```python
from build123d import *

# Parameters (mm, degrees)
SKETCH1_W               = 212.5
SKETCH1_H               = 339.725
BOSS_EXTRUDE1_DEPTH     = 6
SKETCH2_W               = 6.5
SKETCH2_H               = 20
BOSS_EXTRUDE2_DEPTH     = 24
CUT_EXTRUDE1_DEPTH      = 393.36344838
CUT_EXTRUDE1_DEPTH_BACK = 393.36344838
SKETCH3_R               = 4
FILLET2_R               = 5
SKETCH5_R               = 3.175
CUT_EXTRUDE2_DEPTH      = 402.314497153


with BuildPart() as part:
    # Sketch1 → Boss-Extrude1 (new body)
    with BuildSketch(Plane.XY):
        with Locations((106.25, -169.8625)):
            Rectangle(SKETCH1_W, SKETCH1_H)
    extrude(amount=BOSS_EXTRUDE1_DEPTH)

    # Sketch2 → Boss-Extrude2 (add)
    with BuildSketch(Plane.XY.offset(6)):
        with Locations((21.75, -35.2425)):
            Rectangle(SKETCH2_W, SKETCH2_H)
        with Locations((50.75, -35.2425)):
            Rectangle(SKETCH2_W, SKETCH2_H)
        with Locations((190.75, -35.2425)):
            Rectangle(SKETCH2_W, SKETCH2_H)
        with Locations((161.75, -35.2425)):
            Rectangle(SKETCH2_W, SKETCH2_H)
        with Locations((133.75, -104.5325)):
            Rectangle(SKETCH2_W, SKETCH2_H)
        with Locations((165.25, -104.5325)):
            Rectangle(SKETCH2_W, SKETCH2_H)
        with Locations((165.25, -235.1925)):
            Rectangle(SKETCH2_W, SKETCH2_H)
        with Locations((21.75, -304.4825)):
            Rectangle(SKETCH2_W, SKETCH2_H)
        with Locations((50.75, -304.4825)):
            Rectangle(SKETCH2_W, SKETCH2_H)
        with Locations((190.75, -304.4825)):
            Rectangle(SKETCH2_W, SKETCH2_H)
        with Locations((161.75, -304.4825)):
            Rectangle(SKETCH2_W, SKETCH2_H)
        with Locations((133.75, -235.1925)):
            Rectangle(SKETCH2_W, SKETCH2_H)
    extrude(amount=BOSS_EXTRUDE2_DEPTH)

    # Sketch3 → Cut-Extrude1 (cut, two sides: drawn at the far end of the back side and taken through both)
    with BuildSketch(Plane.ZY.offset(-18.5).offset(-CUT_EXTRUDE1_DEPTH_BACK)):
        with Locations(Location((18, -35.2425, 0), (0, 0, 180))):
            Circle(SKETCH3_R)
        with Locations((18, -235.1925)):
            Circle(SKETCH3_R)
        with Locations(Location((18, -304.4825, 0), (0, 0, 270))):
            Circle(SKETCH3_R)
        with Locations(Location((18, -104.5325, 0), (0, 0, 180))):
            Circle(SKETCH3_R)
        with BuildLine():
            Line((18, -25.2425), (18, -12.982943413))
            Line((18, -12.982943413), (51.949532367, -12.982943413))
            Line((51.949532367, -12.982943413), (51.949532367, -57.481006387))
            Line((51.949532367, -57.481006387), (18, -57.481006387))
            Line((18, -57.481006387), (18, -45.2425))
            ThreePointArc((18, -45.2425), (28, -35.2425), (18, -25.2425))
        make_face()
        with BuildLine():
            Line((52.442304634, -132.399123951), (18, -132.399123951))
            Line((18, -132.399123951), (18, -114.5325))
            ThreePointArc((18, -114.5325), (28, -104.5325), (18, -94.5325))
            Line((18, -94.5325), (18, -71.59149594))
            Line((18, -71.59149594), (52.442304634, -71.59149594))
            Line((52.442304634, -71.59149594), (52.442304634, -132.399123951))
        make_face()
        with BuildLine():
            Line((52.599532243, -270.375386727), (18, -270.375386727))
            Line((18, -270.375386727), (18, -245.1925))
            ThreePointArc((18, -245.1925), (28, -235.1925), (18, -225.1925))
            Line((18, -225.1925), (18, -207.306351849))
            Line((18, -207.306351849), (52.599532243, -207.306351849))
            Line((52.599532243, -207.306351849), (52.599532243, -270.375386727))
        make_face()
        with BuildLine():
            Line((52.621034016, -326.721115515), (18, -326.721115515))
            Line((18, -326.721115515), (18, -314.4825))
            ThreePointArc((18, -314.4825), (28, -304.4825), (18, -294.4825))
            Line((18, -294.4825), (18, -282.222834285))
            Line((18, -282.222834285), (52.621034016, -282.222834285))
            Line((52.621034016, -282.222834285), (52.621034016, -326.721115515))
        make_face()
    extrude(amount=CUT_EXTRUDE1_DEPTH + CUT_EXTRUDE1_DEPTH_BACK, mode=Mode.SUBTRACT)

    # Fillet2
    fillet2_edges = [part.edges().sort_by_distance(p)[0] for p in [
        (190.75, -45.2425, 6),
        (194, -35.2425, 6),
        (190.75, -25.2425, 6),
        (50.75, -45.2425, 6),
        (54, -35.2425, 6),
        (50.75, -25.2425, 6),
        (21.75, -25.2425, 6),
        (18.5, -35.2425, 6),
        (21.75, -45.2425, 6),
        (161.75, -25.2425, 6),
        (158.5, -35.2425, 6),
        (161.75, -45.2425, 6),
        (161.75, -294.4825, 6),
        (161.75, -314.4825, 6),
        (158.5, -304.4825, 6),
        (190.75, -314.4825, 6),
        (194, -304.4825, 6),
        (190.75, -294.4825, 6),
        (165.25, -245.1925, 6),
        (168.5, -235.1925, 6),
        (165.25, -225.1925, 6),
        (133.75, -225.1925, 6),
        (130.5, -235.1925, 6),
        (133.75, -245.1925, 6),
        (50.75, -314.4825, 6),
        (54, -304.4825, 6),
        (50.75, -294.4825, 6),
        (21.75, -294.4825, 6),
        (21.75, -314.4825, 6),
        (18.5, -304.4825, 6),
        (165.25, -114.5325, 6),
        (165.25, -94.5325, 6),
        (168.5, -104.5325, 6),
        (133.75, -94.5325, 6),
        (130.5, -104.5325, 6),
        (133.75, -114.5325, 6),
    ]]
    fillet(fillet2_edges, radius=FILLET2_R)

    # Sketch5 → Cut-Extrude2 (cut, through all)
    with BuildSketch(Plane.XY.offset(6)):
        with BuildLine():
            Line((141, -10), (86.089952747, -10))
            ThreePointArc((86.089952747, -10), (83.699567237, -11.767840789), (84.689838532, -14.571154312))
            Line((84.689838532, -14.571154312), (139.599885785, -51.690714779))
            ThreePointArc((139.599885785, -51.690714779), (142.172543061, -51.827533014), (143.5, -49.619560467))
            Line((143.5, -49.619560467), (143.5, -12.5))
            ThreePointArc((143.5, -12.5), (142.767766953, -10.732233047), (141, -10))
        make_face()
        with BuildLine():
            ThreePointArc((0, -12.7), (3.719743879, -3.719743879), (12.7, 0))
            Line((12.7, 0), (0, 0))
            Line((0, 0), (0, -12.7))
        make_face()
        with BuildLine():
            Line((212.5, 0), (199.8, 0))
            ThreePointArc((199.8, 0), (208.780256121, -3.719743879), (212.5, -12.7))
            Line((212.5, -12.7), (212.5, 0))
        make_face()
        with BuildLine():
            ThreePointArc((5, -70.4825), (1.464466094, -69.018033906), (0, -65.4825))
            Line((0, -65.4825), (0, -274.2425))
            ThreePointArc((0, -274.2425), (1.464466094, -270.706966094), (5, -269.2425))
            Line((5, -269.2425), (101.25, -269.2425))
            ThreePointArc((101.25, -269.2425), (104.785533906, -267.778033906), (106.25, -264.2425))
            Line((106.25, -264.2425), (106.25, -204.9525))
            ThreePointArc((106.25, -204.9525), (107.714466094, -201.416966094), (111.25, -199.9525))
            Line((111.25, -199.9525), (187.26, -199.9525))
            ThreePointArc((187.26, -199.9525), (190.795533906, -198.488033906), (192.26, -194.9525))
            Line((192.26, -194.9525), (192.26, -144.7725))
            ThreePointArc((192.26, -144.7725), (190.795533906, -141.236966094), (187.26, -139.7725))
            Line((187.26, -139.7725), (111.25, -139.7725))
            ThreePointArc((111.25, -139.7725), (107.714466094, -138.308033906), (106.25, -134.7725))
            Line((106.25, -134.7725), (106.25, -75.4825))
            ThreePointArc((106.25, -75.4825), (104.785533906, -71.946966094), (101.25, -70.4825))
            Line((101.25, -70.4825), (5, -70.4825))
        make_face()
        with BuildLine():
            Line((212.5, -339.725), (212.5, -327.025))
            ThreePointArc((212.5, -327.025), (208.780256121, -336.005256121), (199.8, -339.725))
            Line((199.8, -339.725), (212.5, -339.725))
        make_face()
        with BuildLine():
            Line((0, -339.725), (12.7, -339.725))
            ThreePointArc((12.7, -339.725), (3.719743879, -336.005256121), (0, -327.025))
            Line((0, -327.025), (0, -339.725))
        make_face()
        with BuildLine():
            ThreePointArc((72.900114215, -18.671785221), (70.327456939, -18.534966986), (69, -20.742939533))
            Line((69, -20.742939533), (69, -57.8625))
            ThreePointArc((69, -57.8625), (69.732233047, -59.630266953), (71.5, -60.3625))
            Line((71.5, -60.3625), (126.410047253, -60.3625))
            ThreePointArc((126.410047253, -60.3625), (128.800432763, -58.594659211), (127.810161468, -55.791345688))
            Line((127.810161468, -55.791345688), (72.900114215, -18.671785221))
        make_face()
        with BuildLine():
            Line((126.410047253, -279.3625), (71.5, -279.3625))
            ThreePointArc((71.5, -279.3625), (69.732233047, -280.094733047), (69, -281.8625))
            Line((69, -281.8625), (69, -318.982060467))
            ThreePointArc((69, -318.982060467), (70.327456939, -321.190033014), (72.900114215, -321.053214779))
            Line((72.900114215, -321.053214779), (127.810161468, -283.933654312))
            ThreePointArc((127.810161468, -283.933654312), (128.800432763, -281.130340789), (126.410047253, -279.3625))
        make_face()
        with BuildLine():
            Line((139.599885785, -288.034285221), (84.689838532, -325.153845688))
            ThreePointArc((84.689838532, -325.153845688), (83.699567237, -327.957159211), (86.089952747, -329.725))
            Line((86.089952747, -329.725), (141, -329.725))
            ThreePointArc((141, -329.725), (142.767766953, -328.992766953), (143.5, -327.225))
            Line((143.5, -327.225), (143.5, -290.105439533))
            ThreePointArc((143.5, -290.105439533), (142.172543061, -287.897466986), (139.599885785, -288.034285221))
        make_face()
        with Locations((12.7, -12.7)):
            Circle(SKETCH5_R)
        with Locations((199.8, -12.7)):
            Circle(SKETCH5_R)
        with Locations((12.7, -327.025)):
            Circle(SKETCH5_R)
        with Locations((199.8, -327.025)):
            Circle(SKETCH5_R)
    extrude(amount=-CUT_EXTRUDE2_DEPTH, mode=Mode.SUBTRACT)


solid = part.part
```
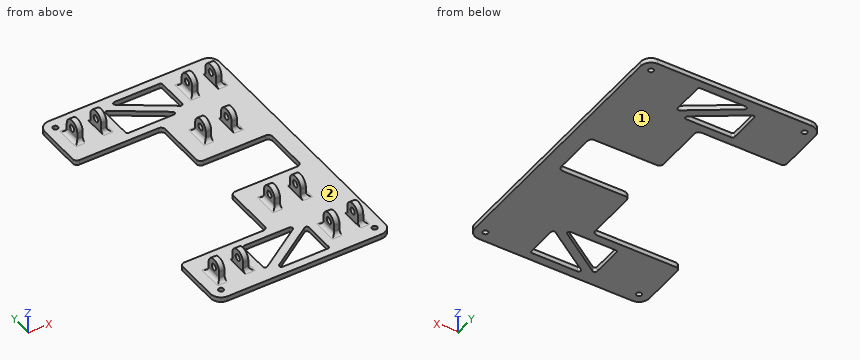
For this review, take the finished solid that the model builds, in its own axes (mm). Face numbers are marked on the shaded views. Round coordinates to 2 decimals unless told otherwise and drop trailing zeros. Write each loop counter-clockwise with the first axis right and the second up, starting at its lowest first coordinate (ties: lowest second). Pieces come first, ordered by that corner, then holes.
1) Take a section at A-A on x = 39.5. Give the boundary of the cut face in (y, z) (1 decimal), then the cut area to 3 significant figures.
Answer below:
outline: (-339.7, 0) - (-269.2, 0) - (-269.2, 6) - (-339.7, 6) - close; (-70.5, 0) - (0, 0) - (0, 6) - (-70.5, 6) - close
area: 846 mm2
2) Take a section at B-B on y = -304. State how many separate pieces and enclosed holes the cut face has, then the cut area to 3 significant figures.
Answer below:
separate pieces: 7
enclosed holes: 0
area: 1,320 mm2
3) Mouldability with a two-part tool opening along X and no side actions: class the marked faces 1 and 2 as +X half, -X half, draft (parallel to the pull), parting line (faces both ways), or undercut.
Answer below:
face 1: draft
face 2: undercut
4) Insertion check: pin 1 Ø2 at (x, z) = (23.5, 15) entering from +Y; pin 2 Ø5 at (x, z) = (163, 14.5) entering from -Y; pin 3 Ø3 at (x, z) = (134, 14) entering from -Y; pin 4 Ø2 at (x, z) = (55.5, 20) entering from -Y. Each pin has a flat end and moves straight along its axis. Give the tip position at first contact, or say it passes through.
Answer below:
pin 1: stops at y = -25.24
pin 2: stops at y = -314.48
pin 3: stops at y = -245.19
pin 4: passes through
5) For line 1 along Y through (x, z) = (166.75, 18); line 2 along Y through (x, z) = (199.8, 2) (3 decimals); line 3 along X through (y, z) = (-299.5, 10), list the stretches that pass through material, from the lowest coordinate up.
Answer below:
line 1: y = -245.19 to -239.19, -231.19 to -225.19, -114.53 to -108.53, -100.53 to -94.53
line 2: y = -339.725 to -330.2, -323.85 to -15.875, -9.525 to 0
line 3: x = 18.4 to 25, 47.5 to 54.1, 158.4 to 165, 187.5 to 194.1
